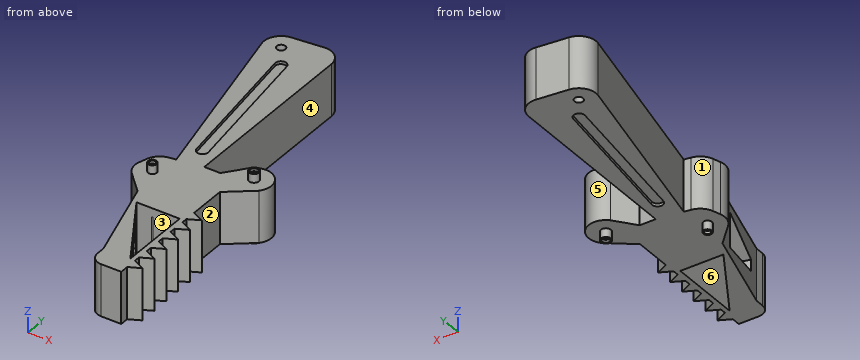
from build123d import *

# Parameters (mm, degrees)
BOSS_EXTRUDE1_DEPTH     = 18
FILLET1_R               = 6
FILLET2_R               = 6
FILLET3_R               = 4
BOSS_EXTRUDE2_DEPTH     = 18
LPATTERN1_COUNT         = 6
LPATTERN1_PITCH         = 6
CUT_EXTRUDE1_DEPTH      = 24
CUT_EXTRUDE2_DEPTH      = 7
CUT_EXTRUDE3_DEPTH      = 1
CUT_EXTRUDE3_DEPTH_BACK = 24
SKETCH5_R               = 1.5
SKETCH6_R               = 1.5
SKETCH6_R_2             = 1.75
BOSS_EXTRUDE3_DEPTH     = 3
SKETCH7_R               = 1
CUT_EXTRUDE4_DEPTH      = 1
SKETCH8_R               = 1.25
CUT_EXTRUDE5_DEPTH      = 1
CUT_EXTRUDE6_DEPTH      = 1


with BuildPart() as part:
    # Sketch1 → Boss-Extrude1 (new body)
    with BuildSketch(Plane.XY):
        Polygon((0, -71), (-8.794264851, -72.38913139), (-24, -2.38913139), (0, 0), align=None)
        with BuildLine():
            ThreePointArc((11, -64.173420673), (19.477467135, -63.809345165), (19.841542643, -72.2868123))
            Line((19.841542643, -72.2868123), (11, -79.141297469))
            Line((11, -79.141297469), (11, -129.141297469))
            Line((11, -129.141297469), (0, -129.141297469))
            Line((0, -129.141297469), (0, -122.141297469))
            Line((0, -122.141297469), (-8.711760915, -92.141297469))
            Line((-8.711760915, -92.141297469), (-17.830063901, -82.875416472))
            Line((-17.830063901, -82.875416472), (-14.816298261, -73.340364471))
            Line((-14.816298261, -73.340364471), (-8.794264851, -72.38913139))
            Line((-8.794264851, -72.38913139), (0, -71))
            Line((0, -71), (5.584872413, -71))
            Line((5.584872413, -71), (11, -64.173420673))
        make_face()
    extrude(amount=BOSS_EXTRUDE1_DEPTH)

    # Fillet1
    fillet1_edges = [part.edges().sort_by_distance(p)[0] for p in [
        (-24, -2.38913139, 9),
        (0, 0, 9),
    ]]
    fillet(fillet1_edges, radius=FILLET1_R)

    # Fillet2
    fillet2_edges = [part.edges().sort_by_distance(p)[0] for p in [
        (-17.830063901, -82.875416472, 9),
        (-14.816298261, -73.340364471, 9),
    ]]
    fillet(fillet2_edges, radius=FILLET2_R)

    # Fillet3
    fillet3_edges = [part.edges().sort_by_distance(p)[0] for p in [
        (0, -129.141297469, 9),
    ]]
    fillet(fillet3_edges, radius=FILLET3_R)

    # Sketch2 → Boss-Extrude2 (add)
    with BuildSketch(Plane(origin=(0, 0, 0), x_dir=(-1, 0, 0), z_dir=(0, 0, -1))):
        Polygon((-11, -126.141297469), (-11, -122.141297469), (-15, -124.141297469), align=None)
    boss_extrude2 = extrude(amount=-BOSS_EXTRUDE2_DEPTH)

    # LPattern1: Boss-Extrude2 ×6
    with Locations(*[(0, i * LPATTERN1_PITCH, 0) for i in range(1, LPATTERN1_COUNT)]):
        add(boss_extrude2)

    # Sketch3 → Cut-Extrude1 (cut)
    with BuildSketch(Plane.XY.offset(18)):
        Polygon((9.307447599, -122.0415562), (9.307447599, -97.0415562), (-5.692552401, -97.0415562), align=None)
    extrude(amount=-CUT_EXTRUDE1_DEPTH, mode=Mode.SUBTRACT)

    # Sketch4 → Cut-Extrude2 (cut)
    with BuildSketch(Plane(origin=(-32.710466491, -9.498858783, 0), x_dir=(0, 0, 1), z_dir=(-0.9603283669964562, -0.2788717044483353, 0))):
        Polygon((3, -93.056438116), (15, -93.056438116), (11, -112.295752741), (7, -112.295752741), align=None)
    extrude(amount=-CUT_EXTRUDE2_DEPTH, mode=Mode.SUBTRACT)

    # Sketch5 → Cut-Extrude3 (cut, two sides: drawn at the far end of the back side and taken through both)
    with BuildSketch(Plane.XY.offset(18).offset(-CUT_EXTRUDE3_DEPTH_BACK)):
        with Locations((-16.707964916, -7.692885756)):
            Circle(SKETCH5_R)
    extrude(amount=CUT_EXTRUDE3_DEPTH + CUT_EXTRUDE3_DEPTH_BACK, mode=Mode.SUBTRACT)

    # Sketch6 → Boss-Extrude3 (add)
    with BuildSketch(Plane.XY.offset(18)):
        with Locations((-11.020793941, -81.240669864)):
            Circle(SKETCH6_R)
        with Locations((15.420771321, -68.230116487)):
            Circle(SKETCH6_R_2)
    boss_extrude3 = extrude(amount=BOSS_EXTRUDE3_DEPTH)

    # Sketch7 → Cut-Extrude4 (cut)
    with BuildSketch(Plane.XY.offset(21)):
        with Locations((-11.020793941, -81.240669864)):
            Circle(SKETCH7_R)
    cut_extrude4 = extrude(amount=-CUT_EXTRUDE4_DEPTH, mode=Mode.SUBTRACT)

    # Sketch8 → Cut-Extrude5 (cut)
    with BuildSketch(Plane.XY.offset(21)):
        with Locations((15.420771321, -68.230116487)):
            Circle(SKETCH8_R)
    cut_extrude5 = extrude(amount=-CUT_EXTRUDE5_DEPTH, mode=Mode.SUBTRACT)

    # Sketch9 → Cut-Extrude6 (cut)
    with BuildSketch(Plane.XY.offset(18)):
        with BuildLine():
            Line((-9.828696114, -14.861442572), (-3.336598594, -64.043999546))
            ThreePointArc((-3.336598594, -64.043999546), (-4.98006279, -66.187319211), (-7.123382455, -64.543855015))
            Line((-7.123382455, -64.543855015), (-13.615479975, -15.361298042))
            ThreePointArc((-13.615479975, -15.361298042), (-11.97201578, -13.217978377), (-9.828696114, -14.861442572))
        make_face()
    cut_extrude6 = extrude(amount=-CUT_EXTRUDE6_DEPTH, mode=Mode.SUBTRACT)

    # Mirror1: Boss-Extrude3, Cut-Extrude4, Cut-Extrude5, Cut-Extrude6 across plane
    add(boss_extrude3.mirror(Plane.XY.offset(9)))
    add(cut_extrude4.mirror(Plane.XY.offset(9)), mode=Mode.SUBTRACT)
    add(cut_extrude5.mirror(Plane.XY.offset(9)), mode=Mode.SUBTRACT)
    add(cut_extrude6.mirror(Plane.XY.offset(9)), mode=Mode.SUBTRACT)


solid = part.part
The listing builds one solid part. Answer for the finished solid, in the listing's coordinates (mm). Face numbers are marked on the shaded views. A direction names the side the tool comes from. Coordinates: 2 decimals unless noted, no trailing zeros. Write each loop counter-clockwise with the first axis right and the second up, starting at its lowest first coordinate (ties: lowest second). Pieces come first, ordered by that corner, then holes. Notation, with made-up numbers: M 37,70 L 62,70 A19 ccw 62,103 Z; hole C 46,32.5 d6. An arc over 180 degrees is marked long. Use one line per item in the form item = value.
Item 1: For the marked faces 1, 2 and 3, determine the directions among +Z, -Z, +X, -X, +Y, -Y from which every point of the face is accessible in a straight line to the end or side of a thin tool.
Model answer:
face_1 = +Z, -Z, -X
face_2 = +Z, -Z, +X
face_3 = +Z, -Z
Item 2: The mould has two halves that part along Y. Classify the marked faces 4, 5 and 6: released by +Y, released by -Y, zero draft, split by the parting line, or undercut.
Model answer:
face_4 = zero draft
face_5 = split by the parting line
face_6 = undercut
Item 3: Given P1, Ø5, axis at x = -9, y = -30, coming from the +Z side; P2, Ø2, axis at y = -103, z = 0, coming from the +X side; P3, Ø8, axis at y = -60.5, z = 14.5, coming from the -X side, each flat-ended and moving along its own axis, determine where each tip first touches the part or whether it passes through.
Model answer:
P1 = 18
P2 = 11.28
P3 = -12.25
Item 4: Find section B-B, the plane y = -53. Give the vertices of the cut face in (x, z).
Model answer:
outline = M -13.01,0 L -8.65,0 L -8.65,1 L -4.79,1 L -4.79,0 L 0,0 L 0,18 L -4.79,18 L -4.79,17 L -8.65,17 L -8.65,18 L -13.01,18 Z
Item 5: Find the intervals of material crossed by probe 1 along Z at (x, y) = (-12, -48.5); probe 2 along Y at (x, z) = (7, 0.25); probe 3 along Z at (x, y) = (-6, -47), in increasing order.
Model answer:
probe_1 = 0 to 18
probe_2 = -129.14 to -118.2, -97.04 to -69.22
probe_3 = 1 to 17
Item 6: Find section C-C, the plane y = -74.5. Give the vertices of the cut face in (x, z), plus the area to 3 significant figures.
Model answer:
outline = M -14.51,0 L 16.99,0 L 16.99,18 L -14.51,18 Z
area = 567 mm2
Item 7: Find section A-A, the plane y = -29. Give the vertices of the cut face in (x, z).
Model answer:
outline = M -18.22,0 L -11.82,0 L -11.82,1 L -7.96,1 L -7.96,0 L 0,0 L 0,18 L -7.96,18 L -7.96,17 L -11.82,17 L -11.82,18 L -18.22,18 Z
